Model file for the job. Use its own axes, mm. Coordinates: 2 decimals unless noted, no trailing zeros. Write each loop counter-clockwise with the first axis right and the second up, starting at its lowest first coordinate (ties: lowest second). Pieces come first, ordered by that corner, then holes.
Q1. Drill centre lines: probe 1 along Z at (x, y) = (1.45, 0) (3 decimals); probe 2 along Y at (x, z) = (1.3, -2.5); probe 3 along Y at (x, z) = (2.5, 1.5). Where is each one in solid material? Low to high.
Q2. Band-saw the part on A-A, the plane x = 1.3. Write the cut outline in (y, z) (3 decimals).
Q3. Pull direction Y, two halves, no side cores. Call faces 1 (the cylindrical face through (2, -3, 0)), 2 (the cylindrical face through (2.94, -3.07, 2.35)): released by +Y, released by -Y, zero draft, split by the parting line, or undercut.
Q4. Pin check, flat tip, straight feed: P1, Ø5, axis at y = 0, z = 0, coming from the -X side. Stop position of the tip, or through.
Autodesk Inventor part; units mm, degrees
ref_plane "YZ Plane" through (0, 0, 0) normal (1, 0, 0) x (0, 1, 0)
ref_plane "XZ Plane" through (0, 0, 0) normal (0, 1, 0) x (-1, 0, 0)
ref_plane "XY Plane" through (0, 0, 0) normal (0, 0, 1) x (1, 0, 0)
sketch "Sketch_58" plane through (0, 0, 0) normal (0, 0, 1) x (1, 0, 0)
  line L0 (50, 0) -> (-50, 0)
  line L1 (0, 3.7983) -> (0, 3.2)
  arc A0 (0, 3.2) -> (0.2, 3) centre (0.2, 3.2) ccw
  line L2 (0.2, 3) -> (3.8, 3)
  arc A1 (3.8, 3) -> (4, 3.2) centre (3.8, 3.2) ccw
  line L3 (4, 3.2) -> (4, 3.7983)
  arc A2 (4, 3.7983) -> (3.9333, 3.865) centre (3.9333, 3.7983) ccw
  line L4 (3.9333, 3.865) -> (2.4767, 3.865)
  arc A3 (1.5233, 3.865) -> (2.4767, 3.865) centre (2, 4.5) ccw
  line L5 (1.5233, 3.865) -> (0.0667, 3.865)
  arc A4 (0.0667, 3.865) -> (0, 3.7983) centre (0.0667, 3.7983) ccw
revolve "Revolution1" add sketch "Sketch_58" angle 360 about axis through (50, 0, 0) along (1, 0, 0)
sketch "Sketch_59" plane through (0, 0, 0) normal (0, 0, 1) x (1, 0, 0)
  line L0 (50, 0) -> (-50, 0)
  line L1 (0, 5.85) -> (0, 3.6)
  line L2 (0, 3.6) -> (0.3812, 3.6)
  arc A0 (0.3812, 3.6) -> (0.582, 3.8008) centre (0.3812, 3.8008) ccw
  line L3 (0.582, 3.8008) -> (0.582, 5.368)
  line L4 (0.582, 5.368) -> (3.418, 5.368)
  line L5 (3.418, 5.368) -> (3.418, 3.8008)
  arc A1 (3.418, 3.8008) -> (3.6188, 3.6) centre (3.6188, 3.8008) ccw
  line L6 (3.6188, 3.6) -> (4, 3.6)
  line L7 (4, 3.6) -> (4, 5.85)
  line L8 (4, 5.85) -> (0, 5.85)
revolve "Revolution2" cut sketch "Sketch_59" angle 360 about axis through (50, 0, 0) along (1, 0, 0)
sketch "Sketch_60" plane through (0, 0, 0) normal (0, 0, 1) x (1, 0, 0)
  line L0 (2, 0) -> (-2, 0)
  line L1 (0.18, 5.45) -> (0.21, 4.9875)
  line L2 (0.21, 4.9875) -> (0.18, 4.525)
  line L3 (0.18, 4.525) -> (0.18, 3.6)
  line L4 (0.18, 3.6) -> (0.24, 3.6)
  line L5 (0.24, 3.6) -> (0.3, 4.525)
  line L6 (0.3, 4.525) -> (0.3, 4.9875)
  line L7 (0.3, 4.9875) -> (0.24, 5.45)
  line L8 (0.24, 5.45) -> (0.18, 5.45)
revolve "Revolution3" add sketch "Sketch_60" angle 360 about axis through (2, 0, 0) along (1, 0, 0)
sketch "Sketch_61" plane through (0, 0, 0) normal (0, 0, 1) x (1, 0, 0)
  line L0 (2, 0) -> (-2, 0)
  line L1 (3.7, 4.525) -> (3.76, 3.6)
  line L2 (3.76, 3.6) -> (3.82, 3.6)
  line L3 (3.82, 3.6) -> (3.82, 4.525)
  line L4 (3.82, 4.525) -> (3.79, 4.9875)
  line L5 (3.79, 4.9875) -> (3.82, 5.45)
  line L6 (3.82, 5.45) -> (3.76, 5.45)
  line L7 (3.76, 5.45) -> (3.7, 4.9875)
  line L8 (3.7, 4.9875) -> (3.7, 4.525)
revolve "Revolution4" add sketch "Sketch_61" angle 360 about axis through (2, 0, 0) along (1, 0, 0)
properties part number "SKF_WBB1-8706-2RS1_PART1"
Answer sheet:
1. probe 1: z = -3.865 to -3, 3 to 3.865
1. probe 2: y = -2.95 to -1.66, 1.66 to 2.95
1. probe 3: y = -3.56 to -2.6, 2.6 to 3.56
2. outline: circle Ø7.73 at (0, 0); hole circle Ø6 at (0, 0)
3. face 1: undercut
3. face 2: split by the parting line
4. P1: passes through
